Can you work these out from the model? Positions are in its coordinate system, mm. Face numbers are marked on the shaded views. Coordinates: 2 decimals unless noted, no trailing zeros. Order: outer loops, then holes, each group sorted by start corner. A loop starts at its lowest first (then second) coordinate and runs counter-clockwise, first axis right, second up. Notation, with made-up numbers: M 54.5,61.5 L 72.5,61.5 A9 ccw 72.5,77.5 Z; hole C -10.75,9.5 d11. An arc over 180 degrees is marked long. Answer as a JSON object with one key per item and string values.
from build123d import *

# Parameters (mm, degrees)
F3_D            = 2
F3_DEPTH        = 4
F3_CBORE_D      = 4.4
F3_CBORE_DEPTH  = 2
F3_TIP          = 0.600860619
F3_COPIES_COUNT = 4


# Not quite as in the source:
# - a pattern or mirror of a feature is missing from the dataset's text; its kind, count and spacing are read off the source's solid


with BuildPart() as f1:
    # F0 (on Front) → F1 (revolve)
    with BuildSketch(Plane.XZ):
        Polygon((-4, 9), (0, 9), (0, 25), (-1, 25), (-4, 22), align=None)
    revolve(axis=Axis((-2, 0, 0), (1, 0, 0)))

    # F3
    with Locations(Plane(origin=(-4, 0, 0), x_dir=(0, -1, 0), z_dir=(-1, 0, 0))):
        with Locations((0, 13)):
            f3 = CounterBoreHole(F3_D / 2, F3_CBORE_D / 2, F3_CBORE_DEPTH, depth=F3_DEPTH)
            with Locations((0, 0, -(F3_DEPTH + F3_TIP / 2))):  # 118° drill point
                Cone(0, F3_D / 2, F3_TIP, mode=Mode.SUBTRACT)

    # F3_copies: F3 ×4 about axis
    f3_copies_axis = Axis((0, 0, 0), (1, 0, 0))
    for i in range(1, F3_COPIES_COUNT):
        add(f3.rotate(f3_copies_axis, i * 360 / F3_COPIES_COUNT), mode=Mode.SUBTRACT)


solid = f1.part
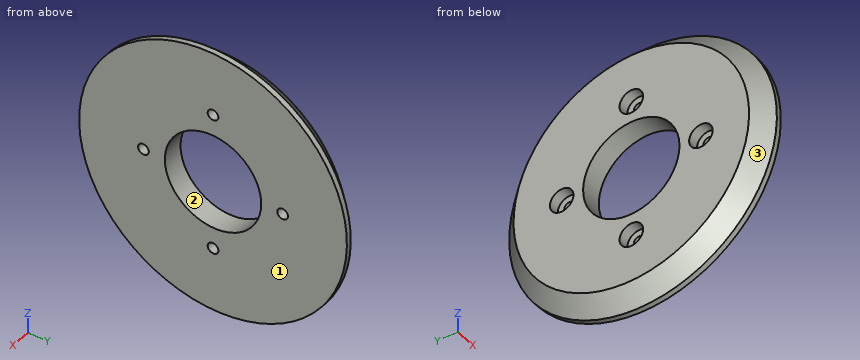
Item 1: If we mould it in two halves opening along Y, with no side actions, what happens to the marked faces 1, 2 and 3? For each: pulls with the +Y half, pulls with the -Y half, needs draft (parallel to the pull), parting line crosses it, or undercut.
Answers follow:
{"face 1": "needs draft", "face 2": "undercut", "face 3": "parting line crosses it"}
Item 2: I want a section at A-A, the plane y = 0. Write out the boundary of the cut face in (x, z).
Answers follow:
{"outline": "M -4,-22 L -1,-25 L 0,-25 L 0,-14 L -2,-14 L -2,-15.2 L -4,-15.2 Z; M -4,-10.8 L -2,-10.8 L -2,-12 L 0,-12 L 0,-9 L -4,-9 Z; M -4,9 L 0,9 L 0,12 L -2,12 L -2,10.8 L -4,10.8 Z; M -4,15.2 L -2,15.2 L -2,14 L 0,14 L 0,25 L -1,25 L -4,22 Z"}
Item 3: Please list where these lines run through material, in increasing order: line 1 (Y direction, x = -0.6, z = 0); line 2 (Z direction, x = -1.2, y = 0); line 3 (Y direction, x = -2.2, z = -0.5).
Answers follow:
{"line 1": "y = -25 to -14, -12 to -9, 9 to 12, 14 to 25", "line 2": "z = -24.8 to -14, -12 to -9, 9 to 12, 14 to 24.8", "line 3": "y = -23.79 to -15.14, -10.86 to -8.99, 8.99 to 10.86, 15.14 to 23.79"}
Item 4: I'm going to push flat-ended pins straight in: pin 1 (1 mm diameter, centred on y = -17.5, z = 16.5, fed in from -X); pin 2 (2.5 mm diameter, centred on y = 0, z = 13, fed in from -X); pin 3 (2 mm diameter, centred on x = -1.5, y = -12, fed in from +Z). Where does each tip first touch, or does it pass through?
Answers follow:
{"pin 1": "stops at x = -2.45", "pin 2": "stops at x = -2", "pin 3": "stops at z = 22.38"}
